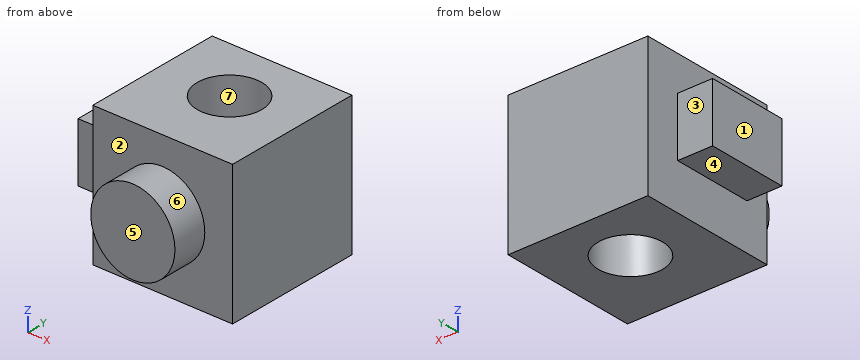
```python
from build123d import *

# Parameters (mm, degrees)
F0_W          = 50.8
F0_H          = 50.8
F0_R          = 15.3727399922
F1_DEPTH      = 50.8
F2_R          = 15.3041702045
F3_DEPTH      = 63.5
F4_W          = 29.5049050776
F4_H          = 21.4435977895
F5_DEPTH      = 12.7
F6_R          = 11.7198726016
F7_DEPTH      = 2540
F7_DEPTH_BACK = 25.4


with BuildPart() as f1:
    # F0 (on Front) → F1 (new body)
    with BuildSketch(Plane.XZ):
        with Locations((25.4, 25.4)):
            Rectangle(F0_W, F0_H)
        with Locations((25.4, 25.4)):
            Circle(F0_R, mode=Mode.SUBTRACT)
        with Locations((25.4, 25.4)):
            Circle(F0_R)
    extrude(amount=F1_DEPTH)

    # F2 (on Front) → F3 (join)
    with BuildSketch(Plane.XZ):
        with Locations((25.4, 25.4)):
            Circle(F2_R)
    extrude(amount=F3_DEPTH)

    # F4 (on face) → F5 (join)
    with BuildSketch(Plane(origin=(0, 0, 0), x_dir=(0, -1, 0), z_dir=(-1, 0, 0))):
        with Locations((27.4524525388, 27.3782011052)):
            Rectangle(F4_W, F4_H)
    extrude(amount=F5_DEPTH)

    # F6 (on face) → F7 (cut, two sides)
    with BuildSketch(Plane.XY.offset(50.8)) as f7_sk:
        with Locations((25.4, -22.3416946828)):
            Circle(F6_R)
    extrude(amount=-F7_DEPTH, mode=Mode.SUBTRACT)
    extrude(f7_sk.sketch, amount=F7_DEPTH_BACK, mode=Mode.SUBTRACT)


solid = f1.part
```
Geometry: final body of the model. Coordinates: model frame, mm. Face numbers are marked on the shaded views. A direction names the side the tool comes from. Round coordinates to 2 decimals unless told otherwise and drop trailing zeros. Write each loop counter-clockwise with the first axis right and the second up, starting at its lowest first coordinate (ties: lowest second). Pieces come first, ordered by that corner, then holes. Notation, with made-up numbers: (-12, -21) -> (41, -21) arc R16 ccw to (41, -17) -> close; hole circle Ø1 at (-22, 63.25). An arc over 180 degrees is marked (long way). Return JSON: item names as keys, results as strings.
Q1. Set-up query: the marked faces 1, 2, 3 and 4. Return all of +Z, -Z, +X, -X, +Y, -Y with unobstructed straight access to the full face (end or side cutting, diameter ignored); none if empty.
From the geometry:
{"face 1": "+Z, -Z, -X, +Y, -Y", "face 2": "-Y", "face 3": "+Z, -Z, -X, +Y", "face 4": "-Z, -X, +Y, -Y"}
Q2. First-contact query: pin 1 Ø6.5 at (x, z) = (-9.5, 24) entering from +Y; pin 2 Ø4 at (x, z) = (-4.5, 31.5) entering from -Y; pin 3 Ø10 at (x, y) = (-5.5, -29.5) entering from +Z. Flat tips, straight axial feed; report the tip coordinate or a pass-through.
From the geometry:
{"pin 1": "y = -12.7", "pin 2": "y = -42.2", "pin 3": "z = 38.1"}
Q3. Mould query, pull axis Y, two halves, no side actions, for the marked faces 5, 6 and 7. Classes: +Y half, -Y half, draft (parallel to the pull), parting line (faces both ways), or undercut.
From the geometry:
{"face 5": "-Y half", "face 6": "draft", "face 7": "undercut"}
Q4. Ray query, line 1 (Y direction, x = 25, z = 31); line 2 (X direction, y = -43.5, z = 16.5); line 3 (Y direction, x = 39.5, z = 12.5). Return the intervals inside material, ascending.
From the geometry:
{"line 1": "-63.5 to -34.05, -10.63 to 0", "line 2": "0 to 50.8", "line 3": "-50.8 to 0"}
Q5. Section C-C on z = 25.4. Return the cut outline in (x, y).
From the geometry:
{"outline": "(-12.7, -42.2) -> (0, -42.2) -> (0, -50.8) -> (10.1, -50.8) -> (10.1, -63.5) -> (40.7, -63.5) -> (40.7, -50.8) -> (50.8, -50.8) -> (50.8, 0) -> (0, 0) -> (0, -12.7) -> (-12.7, -12.7) -> close; hole circle Ø23.44 at (25.4, -22.34)"}
Q6. Section A-A on x = 25.4. Return the cut outline in (y, z).
From the geometry:
{"outline": "(-63.5, 10.1) -> (-50.8, 10.1) -> (-50.8, 0) -> (-34.06, 0) -> (-34.06, 50.8) -> (-50.8, 50.8) -> (-50.8, 40.7) -> (-63.5, 40.7) -> close; (-10.62, 0) -> (0, 0) -> (0, 50.8) -> (-10.62, 50.8) -> close"}
Q7. Section B-B on y = -15.5. Return the cut outline in (x, z).
From the geometry:
{"outline": "(-12.7, 16.66) -> (0, 16.66) -> (0, 0) -> (15.88, 0) -> (15.88, 50.8) -> (0, 50.8) -> (0, 38.1) -> (-12.7, 38.1) -> close; (34.92, 0) -> (50.8, 0) -> (50.8, 50.8) -> (34.92, 50.8) -> close"}
Q8. Section D-D on x = 7.5. Return the cut outline in (y, z), and give its area (3 significant figures).
From the geometry:
{"outline": "(-50.8, 0) -> (0, 0) -> (0, 50.8) -> (-50.8, 50.8) -> close", "area": "2,580 mm2"}
